Study the drawing (mm; zero at the part's minimum x, y, z) and answer. A direction names the side the tool comes from. Coordinates: 2 decimals unless noted, no trailing zeros. Loops run counter-clockwise (first coordinate to the right, second up) from the corner with the lowest first, then second, coordinate; pieces in that order, holes last. Notation, with made-up numbers: (6.5, 60) - (22.5, 60) arc R31 ccw to (22.5, 99) - close; hole circle Ø8 at (-4.75, 2.5). An arc over 180 degrees is marked (long way). Put each result on its own line as item: value.
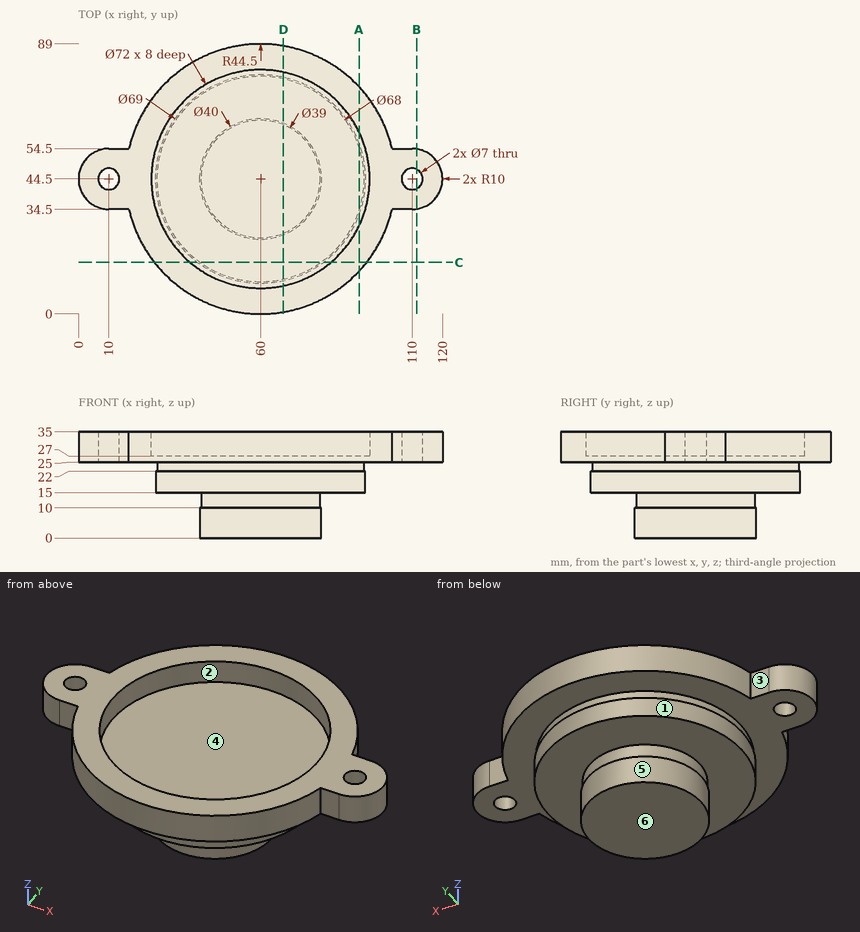
1) The part is cut by section A-A (x = 92.5). Give the vertices of the cut face in (y, z), and give its area (3 significant figures).
Found:
outline: (14.1, 25) - (34.51, 25) - (34.51, 22) - (32.92, 22) - (32.92, 15) - (56.08, 15) - (56.08, 22) - (54.49, 22) - (54.49, 25) - (74.9, 25) - (74.9, 35) - (59.98, 35) - (59.98, 27) - (29.02, 27) - (29.02, 35) - (14.1, 35) - close
area: 582 mm^2
2) For a pull along X with two mould halves and no side action, classify the marked faces 4, 5 and 6 as pulls with the +X half, pulls with the -X half, needs draft (parallel to the pull), parting line crosses it, or undercut.
Found:
face 4: undercut
face 5: parting line crosses it
face 6: needs draft
3) For the marked faces 1, 2 and 3, determine the directions among +Z, -Z, +X, -X, +Y, -Y from which every point of the face is accessible in a straight line to the end or side of a thin tool.
Found:
face 1: -Z
face 2: +Z
face 3: +Z, -Z, -X, +Y
4) The part is cut by section C-C (y = 17). Give the vertices of the cut face in (x, z).
Found:
outline: (25.01, 25) - (40.01, 25) - (40.01, 22) - (39.17, 22) - (39.17, 15) - (80.83, 15) - (80.83, 22) - (79.99, 22) - (79.99, 25) - (94.99, 25) - (94.99, 35) - (83.23, 35) - (83.23, 27) - (36.77, 27) - (36.77, 35) - (25.01, 35) - close
5) The part is cut by section B-B (x = 111.5). Give the vertices of the cut face in (y, z), and give its area (4 significant figures).
Found:
outline: (34.61, 25) - (41.34, 25) - (41.34, 35) - (34.61, 35) - close; (47.66, 25) - (54.39, 25) - (54.39, 35) - (47.66, 35) - close
area: 134.5 mm^2
6) Straight lines are drawn through the part: L1, parallel to Y at x = 10, z = 27.5; L2, parallel to Z at x = 71, y = 30; L3, parallel to X at y = 43, z = 31.5. For each, find the intervals that lie inside material, in ascending order. Write a range as [from, to].
Found:
L1: y = [34.5, 41], [48, 54.5]
L2: z = [0, 27]
L3: x = [0.11, 6.84], [13.16, 24.03], [95.97, 106.84], [113.16, 119.89]
7) Each of these flat-tipped pins is pushed along its axis until it touches: pin 1 (5 mm diameter, centred on x = 40, z = 9.5, fed in from -Y); pin 2 (1.5 mm diameter, centred on y = 23, z = 21.5, fed in from -X); pin 3 (8 mm diameter, centred on x = 10, y = 44.5, fed in from -Z). Where does it stop, or does it pass through?
Found:
pin 1: stops at y = 34.82
pin 2: stops at x = 32.44
pin 3: stops at z = 25
8) The part is cut by section D-D (x = 67.5). Give the vertices of the cut face in (y, z) (1 decimal).
Found:
outline: (0.6, 25) - (11.3, 25) - (11.3, 22) - (10.8, 22) - (10.8, 15) - (26.5, 15) - (26.5, 10) - (26, 10) - (26, 0) - (63, 0) - (63, 10) - (62.5, 10) - (62.5, 15) - (78.2, 15) - (78.2, 22) - (77.7, 22) - (77.7, 25) - (88.4, 25) - (88.4, 35) - (79.7, 35) - (79.7, 27) - (9.3, 27) - (9.3, 35) - (0.6, 35) - close
